Model file for the job. Use its own axes, mm. Face numbers are marked on the shaded views. A direction names the side the tool comes from. Give positions to 0.01 mm unless a question says otherwise; leave off trailing zeros. Order: outer loops, then holes, each group sorted by start corner. A loop starts at its lowest first (then second) coordinate and runs counter-clockwise, first axis right, second up. Notation, with made-up numbers: (42, -20.5) -> (77, -20.5) arc R23 ccw to (77, 8.5) -> close; hole circle Ø7 at (6, 9.25). An arc over 180 degrees is marked (long way). Use CSV: the item, a comma, the result in double quotes. Start each with the question number.
1. Cut at C-C on y = -1.25. List the corners of the cut face in (x, z), then the cut area to 3 significant figures.
2. Wall check: line 1 (X direction, y = 1.55, z = 0); line 2 (Z direction, x = 47.5, y = 0.55); line 3 (X direction, y = -1.1, z = 26). Give the ranges that are in metal, low to high. Write a range as from..to.
3. Cut at A-A on z = 0. List the corners of the cut face in (x, y), then the cut area to 3 significant figures.
4. Pull direction Y, two halves, no side cores. Call the marked faces 3 and 4: released by +Y, released by -Y, zero draft, split by the parting line, or undercut.
5. Cut at B-B on z = 15. List the corners of the cut face in (x, y).
6. Drop flat-ended pins along their axis: pin 1 (2 mm diameter, centred on x = 21, y = -2, fed in from +Z); pin 2 (12 mm diameter, centred on x = -35, z = 15, fed in from -Y); pin 3 (19 mm diameter, centred on x = 4.5, z = 6, fed in from -Y). Give the stop position or say it passes through.
7. 3-axis set-ups, long thin cutter, end or side, ignore diameter. For the marked faces 1 and 2: which of +Z, -Z, +X, -X, +Y, -Y reach the whole face in a straight line?
8. Cut at D-D on x = 12.5. List the corners of the cut face in (y, z).
```python
from build123d import *

# Parameters (mm, degrees)
BOSS_EXTRUDE1_DEPTH  = 2
SKETCH3_R            = 2.05
CUT_EXTRUDE1_DEPTH   = 64.688696014
FILLET1_R            = 5
BOSS_EXTRUDE2_DEPTH  = 5.35
FILLET2_R            = 3.36
FILLET3_R            = 2
FILLET2_OF_MIRROR1_R = 3.36
FILLET3_OF_MIRROR1_R = 2


# Some blends are built 0.0001 mm under size
with BuildPart() as part:
    # Sketch1 → Boss-Extrude1 (new body)
    with BuildSketch(Plane(origin=(0, 0, 0), x_dir=(1, 0, 0), z_dir=(0, 1, 0))):
        Polygon((-52.5, 6), (52.5, 6), (52.5, -6), (30.5, -6), (30.5, -36), (20.5, -36), (20.5, -6), (-20.5, -6), (-20.5, -36), (-30.5, -36), (-30.5, -6), (-52.5, -6), align=None)
    extrude(amount=BOSS_EXTRUDE1_DEPTH)

    # Sketch3 → Cut-Extrude1 (cut, through all)
    with BuildSketch(Plane(origin=(0, 2, 0), x_dir=(1, 0, 0), z_dir=(0, 1, 0))):
        with Locations(Location((-47.5, 0, 0), (0, 0, 270))):
            Circle(SKETCH3_R)
        with Locations(Location((47.5, 0, 0), (0, 0, 90))):
            Circle(SKETCH3_R)
    extrude(amount=-CUT_EXTRUDE1_DEPTH, mode=Mode.SUBTRACT)

    # Fillet1
    fillet1_edges = [part.edges().sort_by_distance(p)[0] for p in [
        (52.5, 1, -6),
        (52.5, 1, 6),
        (20.5, 1, 6),
        (30.5, 1, 6),
        (30.5, 1, 36),
        (20.5, 1, 36),
        (-30.5, 1, 36),
        (-20.5, 1, 36),
        (-20.5, 1, 6),
        (-30.5, 1, 6),
        (-52.5, 1, -6),
        (-52.5, 1, 6),
    ]]
    fillet(fillet1_edges, radius=FILLET1_R - 0.0001)  # a hair under: the kernel refuses the full size

    # Sketch4 → Boss-Extrude2 (add)
    with BuildSketch(Plane(origin=(0, 2, 0), x_dir=(1, 0, 0), z_dir=(0, 1, 0))):
        with BuildLine():
            Line((-20.5, -31), (-20.5, -21))
            Line((-20.5, -21), (-30.5, -21))
            Line((-30.5, -21), (-30.5, -31))
            ThreePointArc((-30.5, -31), (-29.035533906, -34.535533906), (-25.5, -36))
            ThreePointArc((-25.5, -36), (-21.964466094, -34.535533906), (-20.5, -31))
        make_face()
    boss_extrude2 = extrude(amount=-BOSS_EXTRUDE2_DEPTH)

    # Fillet2
    # the kernel refuses this fillet: 3.36 mm, written as the material it adds along each edge
    with BuildSketch(Plane(origin=(-30.5, 0, 21), x_dir=(0, -1, 0), z_dir=(1, 0, 0))) as fillet2_piece_1_section:
        with BuildLine():
            CenterArc((FILLET2_R, FILLET2_R), FILLET2_R, 180, 90)
            Line((0, FILLET2_R), (0, 0))
            Line((0, 0), (FILLET2_R, 0))
        make_face()
    fillet2_piece_1 = extrude(amount=10, mode=Mode.PRIVATE)
    fillet2_piece_1 = split(fillet2_piece_1, bisect_by=Plane(origin=(-25.5, -3.35, 20.239126953), z_dir=(0, 1, 0)), keep=Keep.TOP, mode=Mode.PRIVATE)
    add(fillet2_piece_1)

    # Fillet3
    fillet3_edges = [part.edges().sort_by_distance(p)[0] for p in [
        (-25.5, -3.35, 20.999985119),
    ]]
    fillet(fillet3_edges, radius=FILLET3_R)

    # Mirror1: Boss-Extrude2 across plane
    add(boss_extrude2.mirror(Plane(origin=(0, 0, 0), x_dir=(0, 0, 1), z_dir=(1, 0, 0))))

    # Fillet2 of Mirror1
    # the kernel refuses this fillet: 3.36 mm, written as the material it adds along each edge
    with BuildSketch(Plane(origin=(30.5, 0, 21), x_dir=(0, -1, 0), z_dir=(-1, 0, 0))) as fillet2_of_mirror1_piece_1_section:
        with BuildLine():
            CenterArc((FILLET2_OF_MIRROR1_R, -FILLET2_OF_MIRROR1_R), FILLET2_OF_MIRROR1_R, 90, 90)
            Line((0, -FILLET2_OF_MIRROR1_R), (0, 0))
            Line((0, 0), (FILLET2_OF_MIRROR1_R, 0))
        make_face()
    fillet2_of_mirror1_piece_1 = extrude(amount=10, mode=Mode.PRIVATE)
    fillet2_of_mirror1_piece_1 = split(fillet2_of_mirror1_piece_1, bisect_by=Plane(origin=(25.5, -3.35, 20.239126953), z_dir=(0, 1, 0)), keep=Keep.TOP, mode=Mode.PRIVATE)
    add(fillet2_of_mirror1_piece_1)

    # Fillet3 of Mirror1
    fillet3_of_mirror1_edges = [part.edges().sort_by_distance(p)[0] for p in [
        (25.5, -3.35, 20.999985119),
    ]]
    fillet(fillet3_of_mirror1_edges, radius=FILLET3_OF_MIRROR1_R)


solid = part.part
```
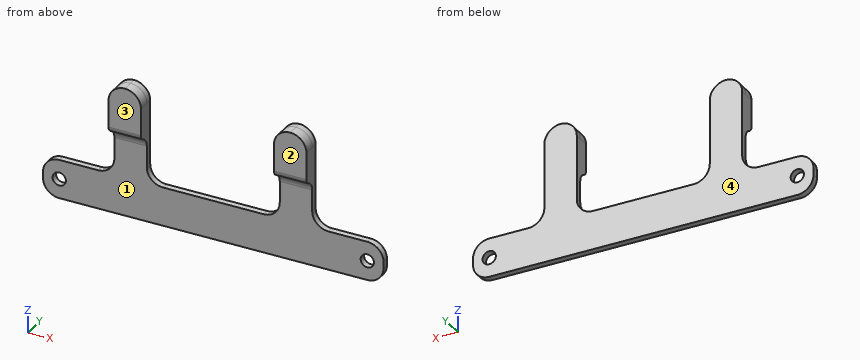
Verdict:
1,outline,"(-30.5, 20.25) -> (-20.5, 20.25) -> (-20.5, 31) arc R5 ccw to (-30.5, 31) -> close; (20.5, 20.25) -> (30.5, 20.25) -> (30.5, 31) arc R5 ccw to (20.5, 31) -> close"
1,area,"293 mm^2"
2,line 1,"-52.5..-49.55, -45.45..45.45, 49.55..52.5"
2,line 2,"-6..-2.05, 2.05..6"
2,line 3,"-30.5..-20.5, 20.5..30.5"
3,outline,"(-52.5, 0) -> (-49.55, 0) -> (-49.55, 2) -> (-52.5, 2) -> close; (-45.45, 0) -> (45.45, 0) -> (45.45, 2) -> (-45.45, 2) -> close; (49.55, 0) -> (52.5, 0) -> (52.5, 2) -> (49.55, 2) -> close"
3,area,"194 mm^2"
4,face 3,"released by -Y"
4,face 4,"released by +Y"
5,outline,"(-30.5, 0) -> (-20.5, 0) -> (-20.5, 2) -> (-30.5, 2) -> close; (20.5, 0) -> (30.5, 0) -> (30.5, 2) -> (20.5, 2) -> close"
6,pin 1,"z = 34.57"
6,pin 2,"y = -0.27"
6,pin 3,"y = 0"
7,face 1,"-Z, +X, -X, -Y"
7,face 2,"+Z, -Z, +X, -X, -Y"
8,outline,"(0, -6) -> (2, -6) -> (2, 6) -> (0, 6) -> close"
